Source: CAD feature listing. Evaluate the final solid. Frame: model axes, mm. Face numbers are marked on the shaded views. A direction names the side the tool comes from. Give positions to 0.01 mm unless a question says otherwise; leave off trailing zeros. Write each loop counter-clockwise with the first axis right and the second up, starting at its lowest first coordinate (ties: lowest second). Pieces come first, ordered by that corner, then holes.
```python
from build123d import *

# Parameters (mm, degrees)
BASPROSKE_W         = 12
BASPROSKE_H         = 20
TOOTHCUT_DEPTH      = 31.724582991
TEETHCUTS_COUNT     = 14
TEETHCUTS_ANGLE     = 334.285714286
BORSKE_R            = 0.4
BORE_DEPTH          = 50.0000508
SKETCH1_R           = 10
BOSS_EXTRUDE1_DEPTH = 10
CUT_EXTRUDE1_START  = -22
CUT_EXTRUDE1_DEPTH  = 22


with BuildPart() as part:
    # BasProSke → Base-Revolve (revolve)
    with BuildSketch(Plane(origin=(0, 0, 0), x_dir=(1, 0, 0), z_dir=(0, 1, 0)), mode=Mode.PRIVATE) as base_revolve_sk:
        with Locations((6, 10)):
            Rectangle(BASPROSKE_W, BASPROSKE_H)
    revolve(base_revolve_sk.sketch.rotate(Axis((-10, 0, 0), (1, 0, 0)), 180), axis=Axis((-10, 0, 0), (1, 0, 0)))

    # TooCutSke → ToothCut (cut, through all)
    with BuildSketch(Plane(origin=(0, 0, 0), x_dir=(0, 0, -1), z_dir=(1, 0, 0))):
        with BuildLine():
            ThreePointArc((1.339503949, 14.311450142), (0, 14.374), (-1.339503949, 14.311450142))
            ThreePointArc((-1.339503949, 14.311450142), (-2.055976555, 17.261705303), (-3.954182827, 19.631125371))
            ThreePointArc((-3.954182827, 19.631125371), (0, 20.0254), (3.954182827, 19.631125371))
            ThreePointArc((3.954182827, 19.631125371), (2.055976555, 17.261705303), (1.339503949, 14.311450142))
        make_face()
    toothcut = extrude(amount=TOOTHCUT_DEPTH, mode=Mode.SUBTRACT)

    # TeethCuts: ToothCut ×14 about axis
    teethcuts_axis = Axis((-10, 0, 0), (1, 0, 0))
    for i in range(1, TEETHCUTS_COUNT):
        add(toothcut.rotate(teethcuts_axis, i * TEETHCUTS_ANGLE / (TEETHCUTS_COUNT - 1)), mode=Mode.SUBTRACT)

    # BorSke → Bore (cut, symmetric)
    with BuildSketch(Plane(origin=(0, 0, 0), x_dir=(0, 0, -1), z_dir=(1, 0, 0))):
        with Locations(Location((0, 0, 0), (0, 0, 180))):
            Circle(BORSKE_R)
    extrude(amount=BORE_DEPTH, both=True, mode=Mode.SUBTRACT)

    # Sketch1 → Boss-Extrude1 (add)
    with BuildSketch(Plane(origin=(12, 0, 0), x_dir=(0, 0, -1), z_dir=(1, 0, 0))):
        with Locations(Location((0, -0.4, 0), (0, 0, 180))):
            Circle(SKETCH1_R)
    extrude(amount=BOSS_EXTRUDE1_DEPTH)

    # Sketch2 → Cut-Extrude1 (cut)
    with BuildSketch(Plane(origin=(22, 0, 0), x_dir=(0, 0, -1), z_dir=(1, 0, 0)).offset(CUT_EXTRUDE1_START)):
        Polygon((6.1, 3.521836642), (0, 7.043673284), (-6.1, 3.521836642), (-6.1, -3.521836642), (0, -7.043673284), (6.1, -3.521836642), align=None)
    extrude(amount=CUT_EXTRUDE1_DEPTH, mode=Mode.SUBTRACT)


solid = part.part
```
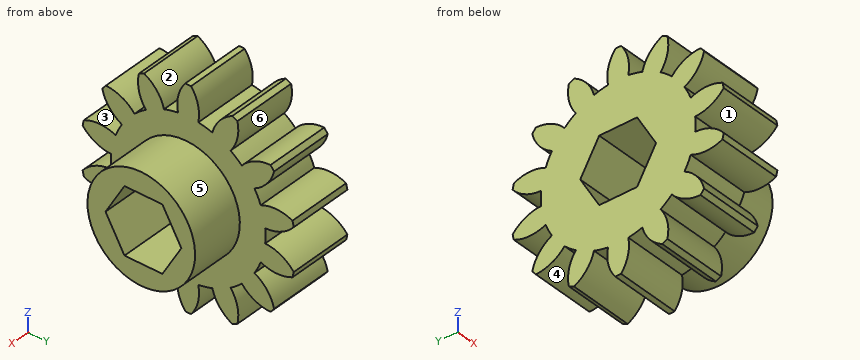
1. Cut plane D-D, the plane z = 9. Return the cut outline in (x, y).
2. Line query: L1, parallel to Z at x = 11.5, y = 0; L2, parallel to Y at x = 9, z = -18; L3, parallel to Z at x = 1.25, y = 15. Output: solid intervals per line, ascending.
3. Access query for the marked faces 1, 2 and 3. Directions: +Z, -Z, +X, -X, +Y, -Y. A direction counts if a zero-diameter tool reaches every point of the face in a straight line with its end or side. Return the directions, or none.
4. Mould query, pull axis Z, two halves, no side actions, for the marked faces 4, 5 and 6. Classes: +Z half, -Z half, draft (parallel to the pull), parting line (faces both ways), or undercut.
5. Cut plane B-B, the plane z = -2. Return the cut outline in (x, y), then the cut area to 3 significant figures.
6. Contact query for flat-ended pins moving along their axis: P1, Ø4, axis at x = 3, y = -7, coming from the -Z side; P2, Ø1, axis at x = 14.5, y = 0.5, coming from the -Z side; P3, Ø5, axis at x = 7, z = -6.5, coming from the +Y side. Output: stop coordinate, or through.
7. Cut plane A-A, the plane x = 19.5. Return the cut outline in (y, z).
8. Cut plane C-C, the plane y = 5. Return the cut outline in (x, z).
Response values:
1. outline: (0, -14.37) - (12, -14.37) - (12, -4.76) - (22, -4.76) - (22, 3.96) - (12, 3.96) - (12, 14.37) - (0, 14.37) - close
2. L1: z = -20 to -6.1, 6.1 to 20
2. L2: y = -8.72 to -7.74, -1.63 to 1.63, 7.74 to 8.72
2. L3: z = -12.87 to -9.81, -5.5 to -1.39, 1.39 to 5.5, 9.81 to 12.87
3. face 1: +X, -X, -Y
3. face 2: +Z, +X, -X
3. face 3: +X, -X
4. face 4: -Z half
4. face 5: parting line
4. face 6: undercut
5. outline: (0, -17.15) - (12, -17.15) - (12, -10.2) - (22, -10.2) - (22, -5.89) - (0, -5.89) - close; (0, 5.89) - (22, 5.89) - (22, 9.4) - (12, 9.4) - (12, 17.15) - (0, 17.15) - close
5. area: 348 mm2
6. P1: stops at z = -18.24
6. P2: stops at z = -9.99
6. P3: stops at y = 19.6
7. outline: circle Ø20 at (-0.4, 0); hole (-7.04, 0) - (-3.52, -6.1) - (3.52, -6.1) - (7.04, 0) - (3.52, 6.1) - (-3.52, 6.1) - close
8. outline: (0, -15.05) - (12, -15.05) - (12, -8.42) - (22, -8.42) - (22, -3.54) - (0, -3.54) - close; (0, 3.54) - (22, 3.54) - (22, 8.42) - (12, 8.42) - (12, 15.05) - (0, 15.05) - close
